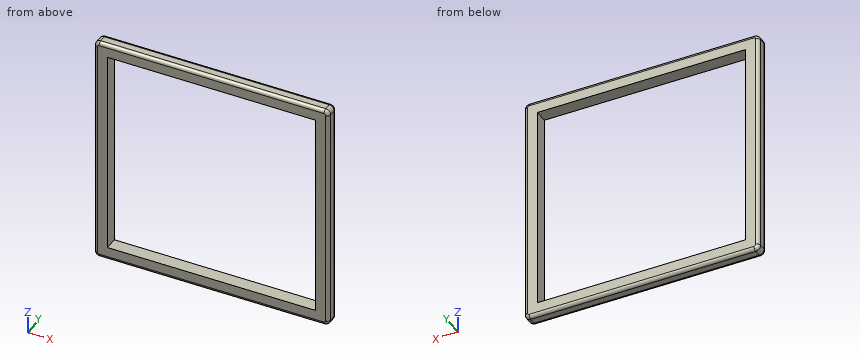
Autodesk Inventor part; units mm, degrees
ref_plane "YZ Plane" through (0, 0, 0) normal (1, 0, 0) x (0, 1, 0)
ref_plane "XZ Plane" through (0, 0, 0) normal (0, 1, 0) x (-1, 0, 0)
ref_plane "XY Plane" through (0, 0, 0) normal (0, 0, 1) x (1, 0, 0)
sketch "Sketch1" plane through (0, 0, 0) normal (0, 1, 0) x (-1, 0, 0)
  line L0 (0, 0) -> (793.75, 0)
  line L1 (793.75, 0) -> (793.75, 793.75)
  line L2 (793.75, 793.75) -> (0, 793.75)
  line L3 (0, 793.75) -> (0, 0)
  line L4 (0, 793.75) -> (793.75, 0) construction
  line L5 (793.75, 793.75) -> (0, 0) construction
  line L6 (844.55, -50.8) -> (-50.8, -50.8)
  line L7 (-50.8, -50.8) -> (-50.8, 844.55)
  line L8 (-50.8, 844.55) -> (844.55, 844.55)
  line L9 (844.55, 844.55) -> (844.55, -50.8)
  line L10 (844.55, -50.8) -> (-50.8, 844.55) construction
  line L11 (-50.8, -50.8) -> (844.55, 844.55) construction
  point P0 (396.875, 396.875)
  dimension "d0" = 793.75
  dimension "d1" = 50.8
  dimension "d2" = 50.8
extrude "Extrusion1" add sketch "Sketch1" along normal blind 50.8
fillet "Fillet1" radius 12.7 8 edges at (-396.875, 50.8, 844.55) (-844.55, 50.8, 396.875) (-396.875, 50.8, -50.8) (50.8, 50.8, 396.875) (-396.875, 0, 844.55) (50.8, 0, 396.875) (-396.875, 0, -50.8) (-844.55, 0, 396.875)
fillet "Fillet2" radius 19.05 12 edges at (47.0803, 47.0803, -47.0803) (47.0803, 3.7197, -47.0803) (50.8, 25.4, -50.8) (47.0803, 47.0803, 840.8303) (47.0803, 3.7197, 840.8303) (50.8, 25.4, 844.55) (-840.8303, 47.0803, 840.8303) (-840.8303, 3.7197, 840.8303) (-844.55, 25.4, 844.55) (-840.8303, 47.0803, -47.0803) (-840.8303, 3.7197, -47.0803) (-844.55, 25.4, -50.8)
properties part number "200555"
Geometry: final body of the model. Coordinates: model frame, mm. Give positions to 0.01 mm unless a question says otherwise; leave off trailing zeros. Write each loop counter-clockwise with the first axis right and the second up, starting at its lowest first coordinate (ties: lowest second). Pieces come first, ordered by that corner, then holes. Notation, with made-up numbers: (2.5, 11) -> (28.5, 11) arc R12 ccw to (28.5, 24) -> close; hole circle Ø7 at (-9, 89.5). An arc over 180 degrees is marked (long way). Answer in a Markdown table with one row per item.
(1) Ray query, line 1 along X through (y, z) = (14, 399); line 2 along X through (y, z) = (39, 444.5); line 3 along Z through (x, y) = (-68, 33). Return the intervals inside material, ascending. Write a range as [from, to].
Answers below:
| item | result |
|---|---|
| line 1 | [-844.55, -793.75], [0, 50.8] |
| line 2 | [-844.52, -793.75], [0, 50.77] |
| line 3 | [-50.8, 0], [793.75, 844.55] |
(2) Pin query (flat end, axial travel): pin 1 (1 mm diameter, centred on y = 39.5, z = 57.5, fed in from -X); pin 2 (3 mm diameter, centred on x = -587, y = 40.5, fed in from +Z); pin 3 (1 mm diameter, centred on x = -567.5, y = 8, fed in from -Z). Return the tip coordinate at first contact, or that it passes through.
Answers below:
| item | result |
|---|---|
| pin 1 | x = -844.52 |
| pin 2 | z = 844.52 |
| pin 3 | z = -50.09 |
(3) Section query C-C on y = 24. Return loops of the section in (x, z).
Answers below:
| item | result |
|---|---|
| outline | (-844.55, -31.75) arc R19.05 ccw to (-825.5, -50.8) -> (31.75, -50.8) arc R19.05 ccw to (50.8, -31.75) -> (50.8, 825.5) arc R19.05 ccw to (31.75, 844.55) -> (-825.5, 844.55) arc R19.05 ccw to (-844.55, 825.5) -> close; hole (-793.75, 0) -> (0, 0) -> (0, 793.75) -> (-793.75, 793.75) -> close |
(4) Section query A-A on x = -228. Return loops of the section in (y, z).
Answers below:
| item | result |
|---|---|
| outline | (0, -38.1) arc R12.7 ccw to (12.7, -50.8) -> (38.1, -50.8) arc R12.7 ccw to (50.8, -38.1) -> (50.8, 0) -> (0, 0) -> close; (0, 793.75) -> (50.8, 793.75) -> (50.8, 831.85) arc R12.7 ccw to (38.1, 844.55) -> (12.7, 844.55) arc R12.7 ccw to (0, 831.85) -> close |
(5) Section query B-B on z = 124. Return loops of the section in (x, y).
Answers below:
| item | result |
|---|---|
| outline | (-844.55, 12.7) arc R12.7 ccw to (-831.85, 0) -> (-793.75, 0) -> (-793.75, 50.8) -> (-831.85, 50.8) arc R12.7 ccw to (-844.55, 38.1) -> close; (0, 0) -> (38.1, 0) arc R12.7 ccw to (50.8, 12.7) -> (50.8, 38.1) arc R12.7 ccw to (38.1, 50.8) -> (0, 50.8) -> close |
